Source: CAD feature listing. Evaluate the final solid. Frame: model axes, mm. A direction names the side the tool comes from. Coordinates: 2 decimals unless noted, no trailing zeros. Write each loop counter-clockwise with the first axis right and the second up, starting at its lowest first coordinate (ties: lowest second). Pieces come first, ordered by that corner, then holes. Notation, with made-up numbers: M 36.5,40.25 L 49.5,40.25 A25 cw 49.5,67.25 Z; hole C 38,75.5 d10. An arc over 180 degrees is marked long. Write item = value, one per line. Start each with the question number.
1. Line query: line 1 along Y through (x, z) = (0, 4); line 2 along Y through (x, z) = (0, 7.5); line 3 along Z through (x, y) = (-2.5, 26.5). Output: solid intervals per line, ascending.
2. Section query B-B (y = 27). Output: boundary loops of the cut face in (x, z), then the cut area to 3 significant figures.
3. Section query C-C (x = 0). Output: boundary loops of the cut face in (y, z), then the cut area to 3 significant figures.
4. Access query for faces 1 (the face through (0, -1, 15)), 2 (the face through (-7.5, 27, 13)), 3 (the face through (28, 0, 20)), 4 (the face through (-22.5, 0, 12)). Directions: +Z, -Z, +X, -X, +Y, -Y. A direction counts if a zero-diameter tool reaches every point of the face in a straight line with its end or side. Return the directions, or none.
5. Pin query (flat end, axial travel): pin 1 Ø6 at (y, z) = (-10.5, 21) entering from -X; pin 2 Ø6 at (x, z) = (23, 14.5) entering from -Y; pin 3 Ø8.5 at (y, z) = (12.5, 20) entering from -X; pin 4 Ø6 at (x, y) = (25.5, -0.5) entering from -Z. Return the tip coordinate at first contact, or that it passes through.
6. Pull-direction query (Z, two-part tool) for faces 5 (the face through (27, 7.5, 13)), 6 (the face through (0, 15, 20)), 7 (the face through (7, -7, 25)), 8 (the face through (0, 0, 10)); classes: pulls with the +Z half, pulls with the -Z half, needs draft (parallel to the pull), parting line crosses it, or undercut.
7. Section query A-A (z = 7). Output: boundary loops of the cut face in (x, y), then the cut area to 3 significant figures.
```python
from build123d import *

# Parameters (mm, degrees)
SKETCH1_R           = 32.5
BOSS_EXTRUDE1_DEPTH = 25
SKETCH2_R           = 20
CUT_EXTRUDE1_DEPTH  = 10
SKETCH3_R           = 7.5
SKETCH3_W           = 30
SKETCH3_H           = 3
SKETCH3_W_2         = 3
SKETCH3_H_2         = 30
CUT_EXTRUDE2_DEPTH  = 10
SKETCH4_W           = 15
SKETCH4_H           = 15
CUT_EXTRUDE3_DEPTH  = 10
SKETCH6_W           = 15
SKETCH6_H           = 15
CUT_EXTRUDE4_DEPTH  = 10
SKETCH7_W           = 15
SKETCH7_H           = 15
CUT_EXTRUDE5_DEPTH  = 10
SKETCH8_W           = 15
SKETCH8_H           = 15
CUT_EXTRUDE6_DEPTH  = 10


with BuildPart() as part:
    # Sketch1 → Boss-Extrude1 (new body)
    with BuildSketch(Plane.XY):
        Circle(SKETCH1_R)
    extrude(amount=BOSS_EXTRUDE1_DEPTH)

    # Sketch2 → Cut-Extrude1 (cut)
    with BuildSketch(Plane(origin=(0, 0, 0), x_dir=(-1, 0, 0), z_dir=(0, 0, -1))):
        Circle(SKETCH2_R)
    extrude(amount=-CUT_EXTRUDE1_DEPTH, mode=Mode.SUBTRACT)

    # Sketch3 → Cut-Extrude2 (cut)
    with BuildSketch(Plane.XY.offset(25)):
        Circle(SKETCH3_R)
        Rectangle(SKETCH3_W, SKETCH3_H)
        Rectangle(SKETCH3_W_2, SKETCH3_H_2)
    extrude(amount=-CUT_EXTRUDE2_DEPTH, mode=Mode.SUBTRACT)

    # Sketch4 → Cut-Extrude3 (cut)
    with BuildSketch(Plane(origin=(32.5, 0, 0), x_dir=(0, 0, -1), z_dir=(1, 0, 0))):
        with Locations((-12.5, 0)):
            Rectangle(SKETCH4_W, SKETCH4_H)
    extrude(amount=-CUT_EXTRUDE3_DEPTH, mode=Mode.SUBTRACT)

    # Sketch6 → Cut-Extrude4 (cut)
    with BuildSketch(Plane.ZY.offset(32.5)):
        with Locations((12.5, 0)):
            Rectangle(SKETCH6_W, SKETCH6_H)
    extrude(amount=-CUT_EXTRUDE4_DEPTH, mode=Mode.SUBTRACT)

    # Sketch7 → Cut-Extrude5 (cut)
    with BuildSketch(Plane(origin=(0, 32.5, 0), x_dir=(1, 0, 0), z_dir=(0, 1, 0))):
        with Locations((0, -12.5)):
            Rectangle(SKETCH7_W, SKETCH7_H)
    extrude(amount=-CUT_EXTRUDE5_DEPTH, mode=Mode.SUBTRACT)

    # Sketch8 → Cut-Extrude6 (cut)
    with BuildSketch(Plane(origin=(0, -32.5, 0), x_dir=(-1, 0, 0), z_dir=(0, -1, 0))):
        with Locations((0, -12.5)):
            Rectangle(SKETCH8_W, SKETCH8_H)
    extrude(amount=-CUT_EXTRUDE6_DEPTH, mode=Mode.SUBTRACT)


solid = part.part
```
Results are:
q1.line_1 = -32.5 to -20, 20 to 32.5
q1.line_2 = -22.5 to -20, 20 to 22.5
q1.line_3 = 0 to 5, 20 to 25
q2.outline = M -18.09,0 L 18.09,0 L 18.09,25 L -18.09,25 Z; hole M -7.5,5 L 7.5,5 L 7.5,20 L -7.5,20 Z
q2.area = 680 mm^2
q3.outline = M -32.5,0 L -20,0 L -20,10 L 20,10 L 20,0 L 32.5,0 L 32.5,5 L 22.5,5 L 22.5,20 L 32.5,20 L 32.5,25 L 15,25 L 15,15 L -15,15 L -15,25 L -32.5,25 L -32.5,20 L -22.5,20 L -22.5,5 L -32.5,5 Z
q3.area = 625 mm^2
q4.face_1 = +Z
q4.face_2 = +Y
q4.face_3 = +X
q4.face_4 = -X
q5.pin_1 = -31.62
q5.pin_2 = -25.62
q5.pin_3 = -31.44
q5.pin_4 = 0
q6.face_5 = undercut
q6.face_6 = needs draft
q6.face_7 = pulls with the +Z half
q6.face_8 = pulls with the -Z half
q7.outline = M -31.62,-7.5 A32.5 ccw -7.5,-31.62 L -7.5,-22.5 L 7.5,-22.5 L 7.5,-31.62 A32.5 ccw 31.62,-7.5 L 22.5,-7.5 L 22.5,7.5 L 31.62,7.5 A32.5 ccw 7.5,31.62 L 7.5,22.5 L -7.5,22.5 L -7.5,31.62 A32.5 ccw -31.62,7.5 L -22.5,7.5 L -22.5,-7.5 Z; hole C 0,0 d40
q7.area = 1,480 mm^2
